The figure shows three views and two pictorial views of one solid part (mm, origin at its lowest corner). Answer the questions. Coordinates: 2 decimals unless noted, no trailing zeros. Loops run counter-clockwise (first coordinate to the right, second up) from the corner with the lowest first, then second, coordinate; pieces in that order, holes last. Notation, with made-up numbers: (-38, 1) - (-8, 1) arc R25 cw to (-8, 24) - close; hole circle Ø5 at (54, 72). An arc over 180 degrees is marked (long way). Write each question's results on one line, items separated by ' | '. Start each with the question number.
Item 1: Section C-C, the plane z = 36 is taken. Write down the section's boundary in (x, y).
Item 2: Section A-A, the plane x = 91.5 is taken. Write down the section's boundary in (y, z) (1 decimal), plus the area to 3 significant figures.
Item 3: This flat-tipped pin is pushed along its axis until it touches: pin 1 Ø2.5 at (x, z) = (155, 5) entering from +Y. Where does it stop, or does it pass through?
Item 4: Consider probe 1 along Z at (x, y) = (155, 0.8); probe 2 along Z at (x, y) = (62.5, 1.8) (1 decimal); probe 3 along X at (y, z) = (1.4, 34). Determine where each line is inside the solid, lowest interval first. Write a range as [from, to].
Item 5: Section B-B, the plane y = 1.35 is taken. Write down the section's boundary in (x, z) (1 decimal), plus the area to 3 significant figures.
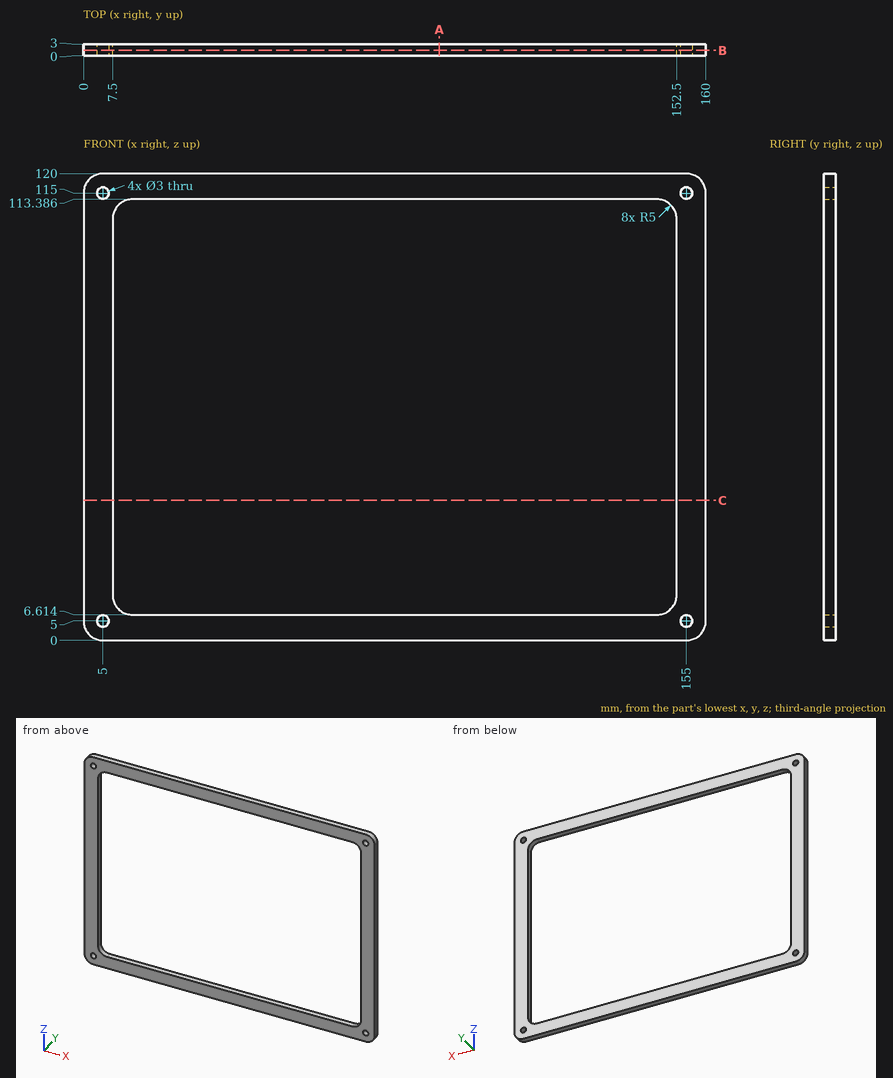
Answer key:
1) outline: (0, 0) - (7.5, 0) - (7.5, 3) - (0, 3) - close; (152.5, 0) - (160, 0) - (160, 3) - (152.5, 3) - close
2) outline: (0, 0) - (3, 0) - (3, 6.6) - (0, 6.6) - close; (0, 113.4) - (3, 113.4) - (3, 120) - (0, 120) - close | area: 39.7 mm^2
3) pin 1: passes through
4) probe 1: z = [0, 3.5], [6.5, 113.5], [116.5, 120] | probe 2: z = [0, 6.6], [113.4, 120] | probe 3: x = [0, 7.5], [152.5, 160]
5) outline: (0, 5) arc R5 ccw to (5, 0) - (155, 0) arc R5 ccw to (160, 5) - (160, 115) arc R5 ccw to (155, 120) - (5, 120) arc R5 ccw to (0, 115) - close; hole circle Ø3 at (5, 5); hole circle Ø3 at (5, 115); hole (7.5, 11.6) arc R5 ccw to (12.5, 6.6) - (147.5, 6.6) arc R5 ccw to (152.5, 11.6) - (152.5, 108.4) arc R5 ccw to (147.5, 113.4) - (12.5, 113.4) arc R5 ccw to (7.5, 108.4) - close; hole circle Ø3 at (155, 5); hole circle Ø3 at (155, 115) | area: 3,690 mm^2
